For this review, take the finished solid that the model builds, in its own axes (mm). A direction names the side the tool comes from. Round coordinates to 2 decimals unless told otherwise and drop trailing zeros. Loops run counter-clockwise (first coordinate to the right, second up) from the corner with the lowest first, then second, coordinate; pieces in that order, holes last. Notation, with made-up numbers: (46.25, 19) -> (64.25, 19) arc R26 ccw to (64.25, 54) -> close; hole circle Ø9 at (-3, -13.5). An arc over 180 degrees is marked (long way). Use one line per item in the form item = value. Start each with the question number.
from build123d import *

# Parameters (mm, degrees)
F0_W        = 35.052
F0_H        = 60.452
F1_DEPTH    = 114.3
F2_R        = 14.0462
F3_DEPTH    = 35.053
F4_R        = 3.175
F5_DEPTH    = 25.4
F6_R        = 9.525
F7_DEPTH    = 114.301
F8_T1_DEPTH = 21.0651495789
F8_T3_DEPTH = 127.3641495789
F8_T5_DEPTH = 126.047561274
F8_T7_DEPTH = 21.0651495789


# Not quite as in the source:
# - a fillet or chamfer that OpenCascade refuses, or shapes differently, is made with other operations: its cross-section is extruded or revolved along the edge and cut away or added


with BuildPart() as f1:
    # F0 (on Front) → F1 (new body)
    with BuildSketch(Plane.XZ):
        Rectangle(F0_W, F0_H)
    extrude(amount=F1_DEPTH)

    # F2 (on face) → F3 (cut, through all)
    with BuildSketch(Plane.YZ.offset(17.526)):
        with Locations((-19.1262, 0)):
            Circle(F2_R)
        with Locations((-50.8762, 0)):
            Circle(F2_R)
        with Locations((-82.6262, 0)):
            Circle(F2_R)
    extrude(amount=-F3_DEPTH, mode=Mode.SUBTRACT)

    # F4 (on face) → F5 (cut)
    with BuildSketch(Plane.XZ.offset(114.3)):
        Circle(F4_R)
    extrude(amount=-F5_DEPTH, mode=Mode.SUBTRACT)

    # F6 (on face) → F7 (cut, through all)
    with BuildSketch(Plane.XZ.offset(114.3)):
        with Locations((0, 30.226)):
            Circle(F6_R)
        with Locations((0, -30.226)):
            Circle(F6_R)
    extrude(amount=-F7_DEPTH, mode=Mode.SUBTRACT)

    # F8: chamfer of 2.54 on 16 edges, made by hand

    # F8_s2 → F8_t1 (cut)
    with BuildSketch(Plane.YZ.offset(-24.0580747894)):
        Polygon((-2.54, 30.226), (0, 27.686), (0, 30.226), align=None)
        Polygon((-111.76, 30.226), (-114.3, 27.686), (-114.3, 30.226), align=None)
        Polygon((0, -27.686), (-2.54, -30.226), (0, -30.226), align=None)
        Polygon((-114.3, -27.686), (-111.76, -30.226), (-114.3, -30.226), align=None)
    extrude(amount=F8_T1_DEPTH, mode=Mode.SUBTRACT)

    # F8_s4 → F8_t3 (cut)
    with BuildSketch(Plane.XZ.offset(-6.5320747894)):
        Polygon((-17.526, 27.686), (-14.986, 30.226), (-17.526, 30.226), align=None)
        Polygon((14.986, 30.226), (17.526, 27.686), (17.526, 30.226), align=None)
        Polygon((-17.526, -27.686), (-14.986, -30.226), (-17.526, -30.226), align=None)
        Polygon((17.526, -27.686), (14.986, -30.226), (17.526, -30.226), align=None)
    extrude(amount=F8_T3_DEPTH, mode=Mode.SUBTRACT)

    # F8_s6 → F8_t5 (cut)
    with BuildSketch(Plane.XZ.offset(-5.873780637)):
        with BuildLine():
            Line((-11.7946015193, 30.226), (-9.3115275153, 28.2207368421))
            ThreePointArc((-9.3115275153, 28.2207368421), (-9.4675743486, 29.181652858), (-9.525, 30.226))
            Line((-9.525, 30.226), (-11.7946015193, 30.226))
        make_face()
        with BuildLine():
            Line((9.3115275153, 28.2207368421), (11.7946015193, 30.226))
            Line((11.7946015193, 30.226), (9.525, 30.226))
            ThreePointArc((9.525, 30.226), (9.4675743486, 29.181652858), (9.3115275153, 28.2207368421))
        make_face()
        with BuildLine():
            Line((-11.7946015193, -30.226), (-9.3115275153, -28.2207368421))
            ThreePointArc((-9.3115275153, -28.2207368421), (-9.4675743486, -29.181652858), (-9.525, -30.226))
            Line((-9.525, -30.226), (-11.7946015193, -30.226))
        make_face()
        with BuildLine():
            Line((11.7946015193, -30.226), (9.3115275153, -28.2207368421))
            ThreePointArc((9.3115275153, -28.2207368421), (9.4675743486, -29.181652858), (9.525, -30.226))
            Line((9.525, -30.226), (11.7946015193, -30.226))
        make_face()
    extrude(amount=F8_T5_DEPTH, mode=Mode.SUBTRACT)

    # F8_s8 → F8_t7 (cut)
    with BuildSketch(Plane.YZ.offset(2.9929252106)):
        Polygon((0, 27.686), (-2.54, 30.226), (0, 30.226), align=None)
        Polygon((-114.3, 27.686), (-111.76, 30.226), (-114.3, 30.226), align=None)
        Polygon((0, -27.686), (-2.54, -30.226), (0, -30.226), align=None)
        Polygon((-114.3, -27.686), (-111.76, -30.226), (-114.3, -30.226), align=None)
    extrude(amount=F8_T7_DEPTH, mode=Mode.SUBTRACT)


solid = f1.part
Item 1: Machinability: for faces 5 (the flat face through (13, -56, -30.226)), 6 (the flat face through (10.536, -56.357, 29.209)), 7 (the flat face through (10.57, -56.357, -29.237)), 8 (the flat face through (13, -56, 30.226)), 9 (the cylindrical face through (-0.69, -105.43, -3.1)), which of the approach directions +Z, -Z, +X, -X, +Y, -Y give a long, thin tool a straight path to every point of the face, cutting with its end or side? Answer none if there is none.
Item 2: Wall thickness on line 1 (Z direction, x = 0, y = -103) (3 decimals); line 2 (X direction, y = -103, z = 0) (3 decimals); line 3 (Y direction, x = 6.5, z = -10): over which ranges is each line inside the solid? List them lowest first.
Item 3: Take a section at D-D on z = -25.5. Give the boundary of the cut face in (x, y).
Item 4: Take a section at B-B on y = -32. Give the boundary of the cut face in (x, z) (3 decimals).
Item 5: Take a section at A-A on z = 0. Give the boundary of the cut face in (x, y) (3 decimals).
Item 6: Draft analysis for pull direction Y (two halves, no side actions). For faces 1 (the flat face through (-4, -114.3, 0)), 2 (the flat face through (-10.57, -56.357, 29.237)), 3 (the flat face through (-13.411, -0.97, -28.656)), 4 (the cylindrical face through (0.25, -64.91, 0.62)), state which applies: +Y half, -Y half, draft (parallel to the pull), parting line (faces both ways), or undercut.
Item 7: Take a section at C-C on x = 0. Give the boundary of the cut face in (y, z) (3 decimals), plus the area to 3 significant figures.
Results:
q1.face_5 = -Z, +X, -X, +Y, -Y
q1.face_6 = +Z, +Y, -Y
q1.face_7 = -Z, +Y, -Y
q1.face_8 = +Z, +X, -X, +Y, -Y
q1.face_9 = -Y
q2.line_1 = -20.701 to -3.175, 3.175 to 20.701
q2.line_2 = -17.526 to -3.175, 3.175 to 17.526
q2.line_3 = -114.3 to -92.49, -72.76 to -60.74, -41.01 to -28.99, -9.26 to 0
q3.outline = (-17.53, -114.3) -> (-8.27, -114.3) -> (-8.27, 0) -> (-17.53, 0) -> close; (8.27, -114.3) -> (17.53, -114.3) -> (17.53, 0) -> (8.27, 0) -> close
q4.outline = (-17.526, -27.686) -> (-14.986, -30.226) -> (-11.795, -30.226) -> (-9.312, -28.221) arc R9.525 cw to (9.312, -28.221) -> (11.795, -30.226) -> (14.986, -30.226) -> (17.526, -27.686) -> (17.526, -5.618) -> (-17.526, -5.618) -> close; (-17.526, 5.618) -> (17.526, 5.618) -> (17.526, 27.686) -> (14.986, 30.226) -> (11.795, 30.226) -> (9.312, 28.221) arc R9.525 cw to (-9.312, 28.221) -> (-11.795, 30.226) -> (-14.986, 30.226) -> (-17.526, 27.686) -> close
q5.outline = (-17.526, -114.3) -> (-3.175, -114.3) -> (-3.175, -96.672) -> (-17.526, -96.672) -> close; (-17.526, -68.58) -> (17.526, -68.58) -> (17.526, -64.922) -> (-17.526, -64.922) -> close; (-17.526, -36.83) -> (17.526, -36.83) -> (17.526, -33.172) -> (-17.526, -33.172) -> close; (-17.526, -5.08) -> (17.526, -5.08) -> (17.526, 0) -> (-17.526, 0) -> close; (3.175, -114.3) -> (17.526, -114.3) -> (17.526, -96.672) -> (3.175, -96.672) -> close
q6.face_1 = -Y half
q6.face_2 = draft
q6.face_3 = +Y half
q6.face_4 = undercut
q7.outline = (-114.3, -20.701) -> (0, -20.701) -> (0, 20.701) -> (-114.3, 20.701) -> (-114.3, 3.175) -> (-96.309, 3.175) arc R14.046 cw (long way) to (-96.309, -3.175) -> (-114.3, -3.175) -> close; hole circle Ø28.092 at (-50.876, 0); hole circle Ø28.092 at (-19.126, 0)
q7.area = 2,760 mm2
